```python
from build123d import *

# Parameters (mm, degrees)
SKETCH1_W                                        = 120
SKETCH1_H                                        = 80
BOSS_EXTRUDE1_DEPTH                              = 7
SKETCH2_W                                        = 110
SKETCH2_H                                        = 70
CUT_EXTRUDE1_DEPTH                               = 3
F_2_6_2_6_DIAMETER_HOLE1_D                       = 2.6
F_2_6_2_6_DIAMETER_HOLE1_DEPTH                   = 4
F_10_2_10_2_DIAMETER_HOLE1_D                     = 10.2
F_10_2_10_2_DIAMETER_HOLE1_DEPTH                 = 4
CBORE_FOR_M2_HEX_HEAD_MACHINE_SCREW1_D           = 2.6
CBORE_FOR_M2_HEX_HEAD_MACHINE_SCREW1_DEPTH       = 7
CBORE_FOR_M2_HEX_HEAD_MACHINE_SCREW1_CBORE_D     = 5
CBORE_FOR_M2_HEX_HEAD_MACHINE_SCREW1_CBORE_DEPTH = 1.5
FILLET1_R                                        = 10
FILLET2_R                                        = 2
FILLET3_R                                        = 5


with BuildPart() as part:
    # Sketch1 → Boss-Extrude1 (new body)
    with BuildSketch(Plane(origin=(0, 7, 0), x_dir=(1, 0, 0), z_dir=(0, 1, 0))):
        Rectangle(SKETCH1_W, SKETCH1_H)
    extrude(amount=-BOSS_EXTRUDE1_DEPTH)

    # Sketch2 → Cut-Extrude1 (cut)
    with BuildSketch(Plane(origin=(0, 7, 0), x_dir=(-1, 0, 0), z_dir=(0, 1, 0))):
        Rectangle(SKETCH2_W, SKETCH2_H)
    extrude(amount=-CUT_EXTRUDE1_DEPTH, mode=Mode.SUBTRACT)

    # Ø2.6 (2.6) Diameter Hole1
    with Locations(Plane(origin=(0, 4, 0), x_dir=(1, 0, 0), z_dir=(0, 1, 0))):
        with Locations((-38, -11), (0, 11), (-11.221825407, -7.778174593), (-19, -11), (-26.778174593, -7.778174593), (-26.778174593, 7.778174593), (-19, 11), (-11.221825407, 7.778174593), (11.221825407, 7.778174593), (19, 11), (26.778174593, 7.778174593), (30, 0), (26.778174593, -7.778174593), (19, -11), (11.221825407, -7.778174593), (-8, 0)):
            Hole(F_2_6_2_6_DIAMETER_HOLE1_D / 2, depth=F_2_6_2_6_DIAMETER_HOLE1_DEPTH)

    # Ø10.2 (10.2) Diameter Hole1
    with Locations(Plane(origin=(0, 4, 0), x_dir=(1, 0, 0), z_dir=(0, 1, 0))):
        with Locations((19, 0), (-19, 0)):
            Hole(F_10_2_10_2_DIAMETER_HOLE1_D / 2, depth=F_10_2_10_2_DIAMETER_HOLE1_DEPTH)

    # CBORE for M2 Hex Head Machine Screw1
    with Locations(Plane(origin=(0, 0, 0), x_dir=(-1, 0, 0), z_dir=(0, -1, 0))):
        with Locations((-8, 0), (30, 0), (38, 11), (-38, 11), (0, -11), (-38, -11)):
            CounterBoreHole(CBORE_FOR_M2_HEX_HEAD_MACHINE_SCREW1_D / 2, CBORE_FOR_M2_HEX_HEAD_MACHINE_SCREW1_CBORE_D / 2, CBORE_FOR_M2_HEX_HEAD_MACHINE_SCREW1_CBORE_DEPTH, depth=CBORE_FOR_M2_HEX_HEAD_MACHINE_SCREW1_DEPTH)

    # Fillet1
    fillet1_edges = [part.edges().sort_by_distance(p)[0] for p in [
        (-60, 3.5, -40),
        (60, 3.5, -40),
        (60, 3.5, 40),
        (-60, 3.5, 40),
    ]]
    fillet(fillet1_edges, radius=FILLET1_R)

    # Fillet2
    fillet2_edges = [part.edges().sort_by_distance(p)[0] for p in [
        (-60, 0, 0),
        (0, 0, 40),
        (0, 0, -40),
        (60, 0, 0),
        (57.071067812, 0, 37.071067812),
        (57.071067812, 0, -37.071067812),
        (-57.071067812, 0, -37.071067812),
        (-57.071067812, 0, 37.071067812),
    ]]
    fillet(fillet2_edges, radius=FILLET2_R)

    # Fillet3
    fillet3_edges = [part.edges().sort_by_distance(p)[0] for p in [
        (-55, 5.5, 35),
        (-55, 5.5, -35),
        (55, 5.5, -35),
        (55, 5.5, 35),
    ]]
    fillet(fillet3_edges, radius=FILLET3_R)


solid = part.part
```
Design review of the part built by this model. Coordinates are the model's own, in mm. A direction names the side the tool comes from. Round coordinates to 2 decimals unless told otherwise and drop trailing zeros. Write each loop counter-clockwise with the first axis right and the second up, starting at its lowest first coordinate (ties: lowest second). Pieces come first, ordered by that corner, then holes.
Item 1: We need section C-C on y = 5.25. Write out the cut boundary in (x, z), and give its area (3 significant figures).
Item 2: We need section D-D on x = -44. Write out the cut boundary in (y, z), and give its area (3 significant figures).
Item 3: Clearance check with flat-ended pins moving along their axes: pin 1 Ø4 at (x, z) = (38, 11) entering from -Y; pin 2 Ø1.5 at (y, z) = (1, 1) entering from -X; pin 3 Ø3 at (x, z) = (19, -11) entering from +Y. State where each tip first meets the part, or that it passes through.
Item 4: We need section A-A on x = 0. Write out the cut boundary in (y, z).
Item 5: For faces 1 (the cylindrical face through (-57.15, 4.46, -36.99)), 2 (the flat face through (55, 6, 0)), 3 (the flat face through (-1.1, 1.5, 12.1)), list the 3-axis set-ups (+Z, -Z, +X, -X, +Y, -Y) from which the entire face can be reached by the end or side of a thin tool; tool diameter is ignored.
Item 6: For probe 1 along Z at (x, y) = (-38, 2.95); probe 2 along Z at (x, y) = (19, 3.2); probe 3 along Z at (x, y) = (-45, 5.25), list the stretches that pass through material, from the lowest coordinate up.
Item 7: The part is to be moulded in two halves that separate along Z. For faces 4 (the flat face through (-1, 5, -40)), 5 (the cylindrical face through (-31.3, 2.77, -0.06)), 6 (the cylindrical face through (10.02, 1.97, -7.28)), 7 (the cylindrical face through (56.99, 4.46, 37.15)), say which applies: +Z half, -Z half, draft (parallel to the pull), parting line (faces both ways), or undercut.
Item 8: We need section B-B on x = -19. Write out the cut boundary in (y, z).
Returned:
1. outline: (-60, -30) arc R10 ccw to (-50, -40) - (50, -40) arc R10 ccw to (60, -30) - (60, 30) arc R10 ccw to (50, 40) - (-50, 40) arc R10 ccw to (-60, 30) - close; hole (-55, -30) arc R5 ccw to (-50, -35) - (50, -35) arc R5 ccw to (55, -30) - (55, 30) arc R5 ccw to (50, 35) - (-50, 35) arc R5 ccw to (-55, 30) - close
1. area: 1,840 mm2
2. outline: (0, -38) arc R2 ccw to (2, -40) - (7, -40) - (7, -35) - (4, -35) - (4, 35) - (7, 35) - (7, 40) - (2, 40) arc R2 ccw to (0, 38) - close
2. area: 348 mm2
3. pin 1: stops at y = 1.5
3. pin 2: stops at x = -59.98
3. pin 3: stops at y = 4
4. outline: (0, -38) arc R2 ccw to (2, -40) - (7, -40) - (7, -35) - (4, -35) - (4, -12.3) - (0, -12.3) - close; (0, -9.7) - (4, -9.7) - (4, 9.7) - (1.5, 9.7) - (1.5, 8.5) - (0, 8.5) - close; (0, 13.5) - (1.5, 13.5) - (1.5, 12.3) - (4, 12.3) - (4, 35) - (7, 35) - (7, 40) - (2, 40) arc R2 ccw to (0, 38) - close
5. face 1: -Z, -X, +Y, -Y
5. face 2: +Y
5. face 3: -Y
6. probe 1: z = -40 to -12.3, -9.7 to 9.7, 12.3 to 40
6. probe 2: z = -40 to -12.3, -9.7 to -5.1, 5.1 to 9.7, 12.3 to 40
6. probe 3: z = -40 to -35, 35 to 40
7. face 4: -Z half
7. face 5: undercut
7. face 6: undercut
7. face 7: +Z half
8. outline: (0, -38) arc R2 ccw to (2, -40) - (7, -40) - (7, -35) - (4, -35) - (4, -12.3) - (0, -12.3) - close; (0, -9.7) - (4, -9.7) - (4, -5.1) - (0, -5.1) - close; (0, 5.1) - (4, 5.1) - (4, 9.7) - (0, 9.7) - close; (0, 12.3) - (4, 12.3) - (4, 35) - (7, 35) - (7, 40) - (2, 40) arc R2 ccw to (0, 38) - close
